Verification items for the finished model (mm, model axes). Round coordinates to 2 decimals unless told otherwise and drop trailing zeros. Order: outer loops, then holes, each group sorted by start corner. A loop starts at its lowest first (then second) coordinate and runs counter-clockwise, first axis right, second up. Notation, with made-up numbers: (67, -37.5) -> (120, -37.5) arc R13 ccw to (120, -32.5) -> close; hole circle Ø8 at (44, 44). An arc over 180 degrees is marked (long way). Answer in a Markdown table with one row per item. Add a question column.
```python
from build123d import *

# Parameters (mm, degrees)
SKETCH1_W               = 6.35
SKETCH1_H               = 38.1
BOSS_EXTRUDE1_DEPTH     = 155.575
F_1_4_CLEARANCE_HOLE1_D = 6.5278


with BuildPart() as part:
    # Sketch1 → Boss-Extrude1 (new, symmetric)
    with BuildSketch(Plane.XY):
        Rectangle(SKETCH1_W, SKETCH1_H)
    extrude(amount=BOSS_EXTRUDE1_DEPTH, both=True)

    # 1/4 Clearance Hole1 (through all)
    with Locations(Plane(origin=(3.175, 0, 0), x_dir=(0, 0, -1), z_dir=(1, 0, 0))):
        with Locations((-147.6375, 0), (-90.4875, 0), (90.4875, 0), (147.6375, 0), (0, 12.7), (0, -12.7)):
            Hole(F_1_4_CLEARANCE_HOLE1_D / 2)


solid = part.part
```
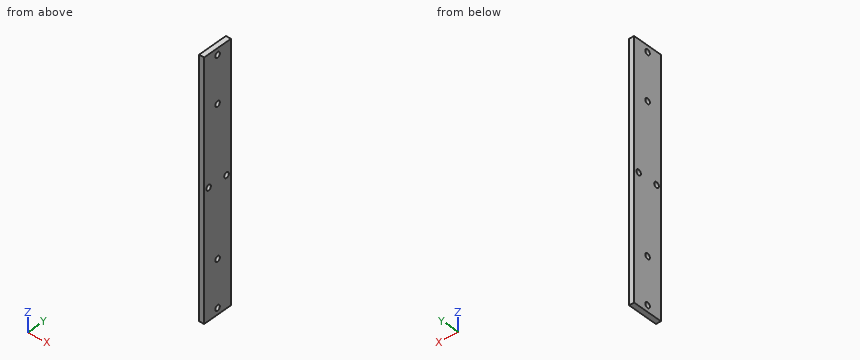
1) Cross-section at D-D, the plane y = 0. Record the boundary of the cut face in (x, z) (3 decimals), and give its area (3 significant figures).
2) Thickness scan on L1, parallel to Y at x = 0.5, z = 0; L2, parallel to Z at x = 2.75, y = 12.5 (3 decimals); L3, parallel to Z at x = -2.5, y = -3 (3 decimals). Record the ranges inside material, lowest first. Write a range as [from, to].
3) Cross-section at A-A, the plane z = 0. Record the boundary of the cut face in (x, y) (3 decimals).
4) Cross-section at C-C, the plane y = -12.7. Record the boundary of the cut face in (x, z) (3 decimals), and give its area (3 significant figures).
5) Cross-section at B-B, the plane x = 0.25. Give the number of separate pieces and of enclosed holes in the cut face, and give its area (3 significant figures).
6) Depth check by flat-ended pin: P1, Ø6, axis at y = -12.7, z = 0, coming from the -X side. Enter the tip coordinate at first touch or a pass-through.
Results below:
| question | item | result |
|---|---|---|
| 1 | outline | (-3.175, -155.575) -> (3.175, -155.575) -> (3.175, -150.901) -> (-3.175, -150.901) -> close; (-3.175, -144.374) -> (3.175, -144.374) -> (3.175, -93.751) -> (-3.175, -93.751) -> close; (-3.175, -87.224) -> (3.175, -87.224) -> (3.175, 87.224) -> (-3.175, 87.224) -> close; (-3.175, 93.751) -> (3.175, 93.751) -> (3.175, 144.374) -> (-3.175, 144.374) -> close; (-3.175, 150.901) -> (3.175, 150.901) -> (3.175, 155.575) -> (-3.175, 155.575) -> close |
| 1 | area | 1,810 mm² |
| 2 | L1 | [-19.05, -15.96], [-9.44, 9.44], [15.96, 19.05] |
| 2 | L2 | [-155.575, -3.258], [3.258, 155.575] |
| 2 | L3 | [-155.575, -148.923], [-146.352, -91.773], [-89.202, 89.202], [91.773, 146.352], [148.923, 155.575] |
| 3 | outline | (-3.175, -19.05) -> (3.175, -19.05) -> (3.175, -15.964) -> (-3.175, -15.964) -> close; (-3.175, -9.436) -> (3.175, -9.436) -> (3.175, 9.436) -> (-3.175, 9.436) -> close; (-3.175, 15.964) -> (3.175, 15.964) -> (3.175, 19.05) -> (-3.175, 19.05) -> close |
| 4 | outline | (-3.175, -155.575) -> (3.175, -155.575) -> (3.175, -3.264) -> (-3.175, -3.264) -> close; (-3.175, 3.264) -> (3.175, 3.264) -> (3.175, 155.575) -> (-3.175, 155.575) -> close |
| 4 | area | 1,930 mm² |
| 5 | separate pieces | 1 |
| 5 | enclosed holes | 6 |
| 5 | area | 11,700 mm² |
| 6 | P1 | through |
